Input: part model. Units: mm. Frame: model coordinates. Round coordinates to 2 decimals unless told otherwise and drop trailing zeros. Loops run counter-clockwise (first coordinate to the right, second up) from the corner with the lowest first, then second, coordinate; pieces in that order, holes last. Notation, with made-up numbers: (21.25, 31) -> (63.25, 31) arc R24 cw to (63.25, 57) -> close; hole circle Ø6 at (71, -25.75). An arc over 180 degrees is marked (long way). Answer in a Markdown table with one row per item. Add a question column.
Q1. Section C-C, the plane x = 3. Output: boundary loops of the cut face in (y, z).
Q2. Section A-A, the plane z = 2.45. Give the number of separate pieces and of enclosed holes in the cut face, and give its area (3 significant figures).
Q3. Ray query, L1, parallel to Y at x = 12, z = 2.3; L2, parallel to Y at x = 51.5, z = 1.9; L3, parallel to Y at x = 104.5, z = 0.7. Return the intervals inside material, ascending. Write a range as from..to.
Q4. Section B-B, the plane y = 59.5. Output: boundary loops of the cut face in (x, z), and give its area (3 significant figures).
Q5. Pin query (flat end, axial travel): pin 1 (2.5 mm diameter, centred on x = 51.5, y = 73, fed in from -Z); pin 2 (1.5 mm diameter, centred on x = 43.5, z = 1, fed in from +Y); pin 3 (1.5 mm diameter, centred on x = 0, z = 1.5, fed in from +Y); pin 4 (0.9 mm diameter, centred on x = -5, z = 2, fed in from -Y). Return the tip coordinate at first contact, or that it passes through.
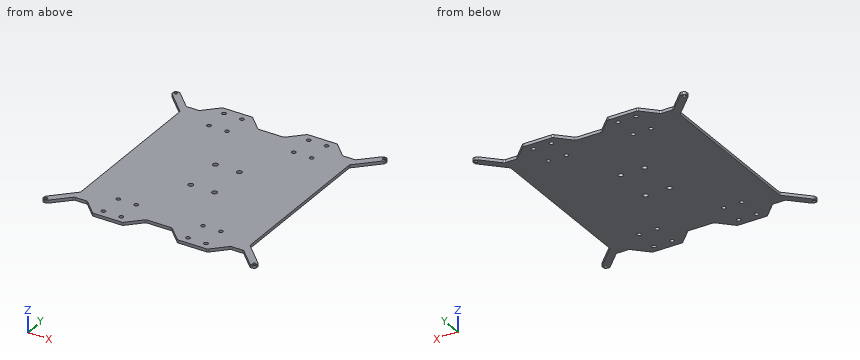
```python
from build123d import *

# Parameters (mm, degrees)
F0_R     = 1.55
F0_R_2   = 2.05
F0_R_3   = 2.55
F1_DEPTH = 3


with BuildPart() as f1:
    # F0 (on Top) → F1 (new body)
    with BuildSketch(Plane.XY):
        with BuildLine():
            Line((-103.035534, 107), (-104.5, 107))
            ThreePointArc((-104.5, 107), (-106.267767, 106.267767), (-107, 104.5))
            Line((-107, 104.5), (-107, 103.035534))
            ThreePointArc((-107, 103.035534), (-106.809699, 102.078825), (-106.267767, 101.267767))
            Line((-106.267767, 101.267767), (-85.732233, 80.732233))
            ThreePointArc((-85.732233, 80.732233), (-85.190301, 79.921175), (-85, 78.964466))
            Line((-85, 78.964466), (-85, -78.964466))
            ThreePointArc((-85, -78.964466), (-85.190301, -79.921175), (-85.732233, -80.732233))
            Line((-85.732233, -80.732233), (-106.267767, -101.267767))
            ThreePointArc((-106.267767, -101.267767), (-106.809699, -102.078825), (-107, -103.035534))
            Line((-107, -103.035534), (-107, -104.5))
            ThreePointArc((-107, -104.5), (-106.267767, -106.267767), (-104.5, -107))
            Line((-104.5, -107), (-103.035534, -107))
            ThreePointArc((-103.035534, -107), (-102.078825, -106.809699), (-101.267767, -106.267767))
            Line((-101.267767, -106.267767), (-85.732233, -90.732233))
            ThreePointArc((-85.732233, -90.732233), (-84.921175, -90.190301), (-83.964466, -90))
            Line((-83.964466, -90), (-73.035534, -90))
            ThreePointArc((-73.035534, -90), (-72.078825, -90.190301), (-71.267767, -90.732233))
            Line((-71.267767, -90.732233), (-58.232233, -103.767767))
            ThreePointArc((-58.232233, -103.767767), (-57.421175, -104.309699), (-56.464466, -104.5))
            Line((-56.464466, -104.5), (-28.535534, -104.5))
            ThreePointArc((-28.535534, -104.5), (-27.578825, -104.309699), (-26.767767, -103.767767))
            Line((-26.767767, -103.767767), (-13.732233, -90.732233))
            ThreePointArc((-13.732233, -90.732233), (-12.921175, -90.190301), (-11.964466, -90))
            Line((-11.964466, -90), (11.964466, -90))
            ThreePointArc((11.964466, -90), (12.921175, -90.190301), (13.732233, -90.732233))
            Line((13.732233, -90.732233), (26.767767, -103.767767))
            ThreePointArc((26.767767, -103.767767), (27.578825, -104.309699), (28.535534, -104.5))
            Line((28.535534, -104.5), (56.464466, -104.5))
            ThreePointArc((56.464466, -104.5), (57.421175, -104.309699), (58.232233, -103.767767))
            Line((58.232233, -103.767767), (71.267767, -90.732233))
            ThreePointArc((71.267767, -90.732233), (72.078825, -90.190301), (73.035534, -90))
            Line((73.035534, -90), (83.964466, -90))
            ThreePointArc((83.964466, -90), (84.921175, -90.190301), (85.732233, -90.732233))
            Line((85.732233, -90.732233), (101.267767, -106.267767))
            ThreePointArc((101.267767, -106.267767), (102.078825, -106.809699), (103.035534, -107))
            Line((103.035534, -107), (104.5, -107))
            ThreePointArc((104.5, -107), (106.267767, -106.267767), (107, -104.5))
            Line((107, -104.5), (107, -103.035534))
            ThreePointArc((107, -103.035534), (106.809699, -102.078825), (106.267767, -101.267767))
            Line((106.267767, -101.267767), (85.732233, -80.732233))
            ThreePointArc((85.732233, -80.732233), (85.190301, -79.921175), (85, -78.964466))
            Line((85, -78.964466), (85, 78.964466))
            ThreePointArc((85, 78.964466), (85.190301, 79.921175), (85.732233, 80.732233))
            Line((85.732233, 80.732233), (106.267767, 101.267767))
            ThreePointArc((106.267767, 101.267767), (106.809699, 102.078825), (107, 103.035534))
            Line((107, 103.035534), (107, 104.5))
            ThreePointArc((107, 104.5), (106.267767, 106.267767), (104.5, 107))
            Line((104.5, 107), (103.035534, 107))
            ThreePointArc((103.035534, 107), (102.078825, 106.809699), (101.267767, 106.267767))
            Line((101.267767, 106.267767), (85.732233, 90.732233))
            ThreePointArc((85.732233, 90.732233), (84.921175, 90.190301), (83.964466, 90))
            Line((83.964466, 90), (73.035534, 90))
            ThreePointArc((73.035534, 90), (72.078825, 90.190301), (71.267767, 90.732233))
            Line((71.267767, 90.732233), (58.232233, 103.767767))
            ThreePointArc((58.232233, 103.767767), (57.421175, 104.309699), (56.464466, 104.5))
            Line((56.464466, 104.5), (28.535534, 104.5))
            ThreePointArc((28.535534, 104.5), (27.578825, 104.309699), (26.767767, 103.767767))
            Line((26.767767, 103.767767), (13.732233, 90.732233))
            ThreePointArc((13.732233, 90.732233), (12.921175, 90.190301), (11.964466, 90))
            Line((11.964466, 90), (-11.964466, 90))
            ThreePointArc((-11.964466, 90), (-12.921175, 90.190301), (-13.732233, 90.732233))
            Line((-13.732233, 90.732233), (-26.767767, 103.767767))
            ThreePointArc((-26.767767, 103.767767), (-27.578825, 104.309699), (-28.535534, 104.5))
            Line((-28.535534, 104.5), (-56.464466, 104.5))
            ThreePointArc((-56.464466, 104.5), (-57.421175, 104.309699), (-58.232233, 103.767767))
            Line((-58.232233, 103.767767), (-71.267767, 90.732233))
            ThreePointArc((-71.267767, 90.732233), (-72.078825, 90.190301), (-73.035534, 90))
            Line((-73.035534, 90), (-83.964466, 90))
            ThreePointArc((-83.964466, 90), (-84.921175, 90.190301), (-85.732233, 90.732233))
            Line((-85.732233, 90.732233), (-101.267767, 106.267767))
            ThreePointArc((-101.267767, 106.267767), (-102.078825, 106.809699), (-103.035534, 107))
        make_face()
        with Locations((-104.5, -104.5)):
            Circle(F0_R, mode=Mode.SUBTRACT)
        with Locations((-51.5, -97)):
            Circle(F0_R_2, mode=Mode.SUBTRACT)
        with Locations((-33.5, -97)):
            Circle(F0_R_2, mode=Mode.SUBTRACT)
        with Locations((-51.5, -73)):
            Circle(F0_R_2, mode=Mode.SUBTRACT)
        with Locations((-33.5, -73)):
            Circle(F0_R_2, mode=Mode.SUBTRACT)
        with Locations((-12, -20)):
            Circle(F0_R_3, mode=Mode.SUBTRACT)
        with Locations((33.5, -97)):
            Circle(F0_R_2, mode=Mode.SUBTRACT)
        with Locations((51.5, -97)):
            Circle(F0_R_2, mode=Mode.SUBTRACT)
        with Locations((33.5, -73)):
            Circle(F0_R_2, mode=Mode.SUBTRACT)
        with Locations((51.5, -73)):
            Circle(F0_R_2, mode=Mode.SUBTRACT)
        with Locations((104.5, -104.5)):
            Circle(F0_R, mode=Mode.SUBTRACT)
        with Locations((12, -20)):
            Circle(F0_R_3, mode=Mode.SUBTRACT)
        with Locations((-12, 20)):
            Circle(F0_R_3, mode=Mode.SUBTRACT)
        with Locations((-104.5, 104.5)):
            Circle(F0_R, mode=Mode.SUBTRACT)
        with Locations((-51.5, 73)):
            Circle(F0_R_2, mode=Mode.SUBTRACT)
        with Locations((-33.5, 73)):
            Circle(F0_R_2, mode=Mode.SUBTRACT)
        with Locations((-51.5, 97)):
            Circle(F0_R_2, mode=Mode.SUBTRACT)
        with Locations((-33.5, 97)):
            Circle(F0_R_2, mode=Mode.SUBTRACT)
        with Locations((12, 20)):
            Circle(F0_R_3, mode=Mode.SUBTRACT)
        with Locations((33.5, 73)):
            Circle(F0_R_2, mode=Mode.SUBTRACT)
        with Locations((51.5, 73)):
            Circle(F0_R_2, mode=Mode.SUBTRACT)
        with Locations((33.5, 97)):
            Circle(F0_R_2, mode=Mode.SUBTRACT)
        with Locations((51.5, 97)):
            Circle(F0_R_2, mode=Mode.SUBTRACT)
        with Locations((104.5, 104.5)):
            Circle(F0_R, mode=Mode.SUBTRACT)
    extrude(amount=F1_DEPTH)


solid = f1.part
```
Answer block:
| question | item | result |
|---|---|---|
| 1 | outline | (-90, 0) -> (90, 0) -> (90, 3) -> (-90, 3) -> close |
| 2 | separate pieces | 1 |
| 2 | enclosed holes | 24 |
| 2 | area | 33,700 mm^2 |
| 3 | L1 | -90..-22.55, -17.45..17.45, 22.55..90 |
| 3 | L2 | -104.5..-99.05, -94.95..-75.05, -70.95..70.95, 75.05..94.95, 99.05..104.5 |
| 3 | L3 | -107..-106.05, -102.95..-99.5, 99.5..102.95, 106.05..107 |
| 4 | outline | (-85, 0) -> (85, 0) -> (85, 3) -> (-85, 3) -> close |
| 4 | area | 510 mm^2 |
| 5 | pin 1 | through |
| 5 | pin 2 | y = 104.5 |
| 5 | pin 3 | y = 90 |
| 5 | pin 4 | y = -90 |
